Answer from the drawing. Dimensions are ordinates in mm from the lowest x, y and z of the part. A direction names the side the tool comes from. Give positions to 0.01 mm unless a question says otherwise; leave off trailing zeros. Loops run counter-clockwise (first coordinate to the right, second up) from the corner with the lowest first, then second, coordinate; pieces in that order, holes last.
(1) Find section B-B, the plane z = 6.5. Write down the section's boundary in (x, y).
(2) Straight lines are drawn through the part: probe 1 along Y at (x, z) = (23, 0.6); probe 2 along Z at (x, y) = (7, 23); probe 3 along X at (y, z) = (15, 13.25). For each, find the intervals that lie inside material, in ascending order.
(3) Find section A-A, the plane y = 3.5. Write down the section's boundary in (x, z), then the cut area to 4 significant figures.
(4) Each of these flat-tipped pins is pushed along its axis until it touches: P1, Ø9, axis at x = 12, y = 15, coming from the +Z side; P2, Ø6, axis at y = 18, z = 8.5, coming from the -X side. Where does it stop, or does it pass through?
(5) Find section C-C, the plane x = 23. Write down the section's boundary in (y, z), then the cut area to 3 significant figures.
(6) Which of the six approach directions +Z, -Z, +X, -X, +Y, -Y give full straight-line access (tool end or side, diameter ignored) to the marked faces 1 and 2?
(7) Find section D-D, the plane y = 27.5. Write down the section's boundary in (x, z).
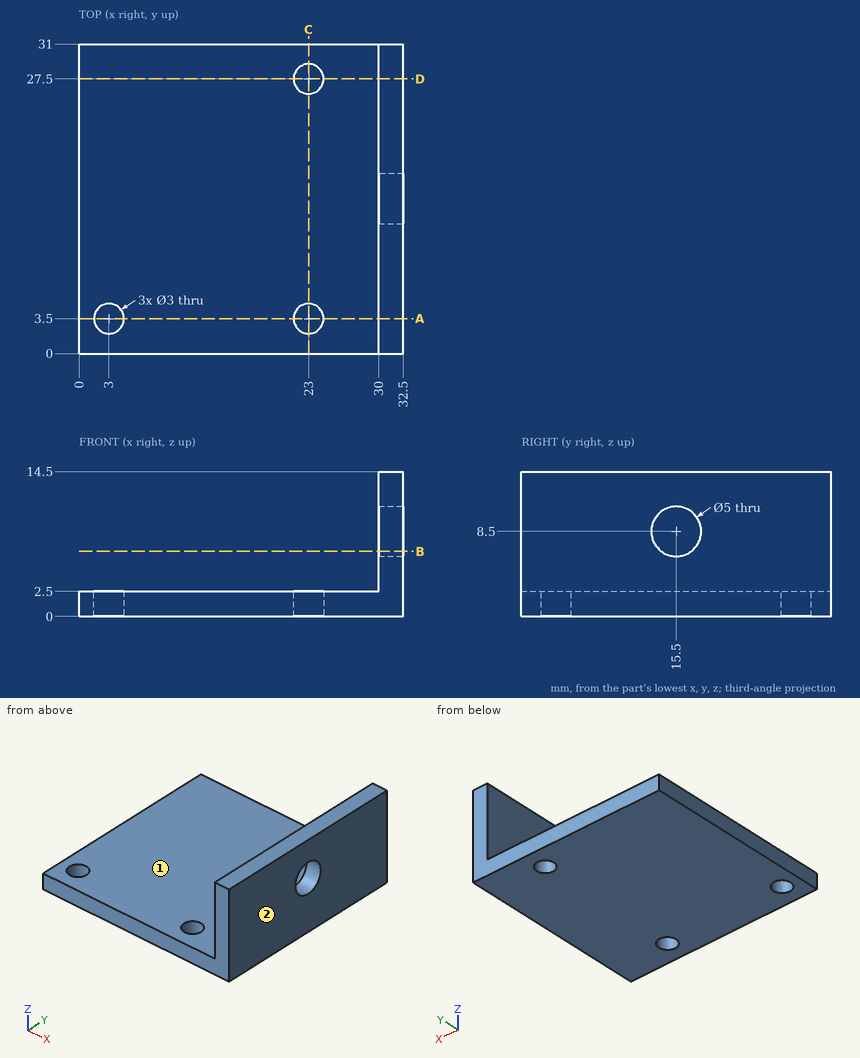
Entries:
1. outline: (30, 0) - (32.5, 0) - (32.5, 14) - (30, 14) - close; (30, 17) - (32.5, 17) - (32.5, 31) - (30, 31) - close
2. probe 1: y = 0 to 2, 5 to 26, 29 to 31
2. probe 2: z = 0 to 2.5
2. probe 3: x = 30 to 32.5
3. outline: (0, 0) - (1.5, 0) - (1.5, 2.5) - (0, 2.5) - close; (4.5, 0) - (21.5, 0) - (21.5, 2.5) - (4.5, 2.5) - close; (24.5, 0) - (32.5, 0) - (32.5, 14.5) - (30, 14.5) - (30, 2.5) - (24.5, 2.5) - close
3. area: 96.25 mm2
4. P1: stops at z = 2.5
4. P2: stops at x = 30
5. outline: (0, 0) - (2, 0) - (2, 2.5) - (0, 2.5) - close; (5, 0) - (26, 0) - (26, 2.5) - (5, 2.5) - close; (29, 0) - (31, 0) - (31, 2.5) - (29, 2.5) - close
5. area: 62.5 mm2
6. face 1: +Z, -X, +Y, -Y
6. face 2: +Z, -Z, +X, +Y, -Y
7. outline: (0, 0) - (21.5, 0) - (21.5, 2.5) - (0, 2.5) - close; (24.5, 0) - (32.5, 0) - (32.5, 14.5) - (30, 14.5) - (30, 2.5) - (24.5, 2.5) - close
